The model under review builds one solid part; all positions refer to its coordinate system, in mm. Give positions to 0.01 mm unless a question says otherwise; leave off trailing zeros. Loops run counter-clockwise (first coordinate to the right, second up) from the corner with the lowest first, then second, coordinate; pieces in that order, holes last. Notation, with made-up numbers: (68, 22.5) - (98, 22.5) arc R19 ccw to (98, 43.5) - close; hole circle Ø5 at (-30, 88). An arc over 180 degrees is marked (long way). Return JSON: item names as keys, results as strings. Group by question number.
```python
from build123d import *

# Parameters (mm, degrees)
BOSS_EXTRUDE1_DEPTH   = 7
F_3_0MM_DOWEL_HOLE1_D = 3


with BuildPart() as part:
    # Sketch1 → Boss-Extrude1 (new body)
    with BuildSketch(Plane.XY):
        with BuildLine():
            ThreePointArc((0, 30), (-30, 0), (0, -30))
            ThreePointArc((0, -30), (5, -25), (0, -20))
            ThreePointArc((0, -20), (-20, 0), (0, 20))
            ThreePointArc((0, 20), (5, 25), (0, 30))
        make_face()
    extrude(amount=BOSS_EXTRUDE1_DEPTH)

    # Ø3.0mm Dowel Hole1 (through all)
    with Locations(Plane.XY.offset(7)):
        with Locations((0, 25), (0, -25)):
            Hole(F_3_0MM_DOWEL_HOLE1_D / 2)


solid = part.part
```
1) We need section D-D, the plane y = 17.5. Write out the cut boundary in (x, z).
2) We need section C-C, the plane y = 25. Write out the cut boundary in (x, z), plus the area to 3 significant figures.
3) For pin 1 Ø1 at (y, z) = (12.5, 4) entering from +X; pin 2 Ø2 at (x, z) = (-6, 6) entering from -Y; pin 3 Ø2 at (y, z) = (3.5, 3.5) entering from +X, all flat-tipped, find the tip position at first contact; note any pin that passes through.
4) We need section A-A, the plane z = 1.5. Write out the cut boundary in (x, y).
5) Draft analysis for pull direction Y (two halves, no side actions). For faces 1 (the face through (-29.993, 0.66, 3.451)), 2 (the face through (-21, 0, 7)), 3 (the face through (-20, 0, 3)), state which applies: +Y half, -Y half, draft (parallel to the pull), parting line (faces both ways), or undercut.
6) To check wall thickness, follow line 1 (Y direction, x = -10, z = 4.5); line 2 (Y direction, x = -16, z = 4.25); line 3 (Y direction, x = -24.5, z = 1). State the ranges of each line that lie inside material, in increasing order.
7) We need section B-B, the plane x = -16. Write out the cut boundary in (y, z).
Findings:
{
 "1": {"outline": "(-24.37, 0) - (-9.68, 0) - (-9.68, 7) - (-24.37, 7) - close"},
 "2": {"outline": "(-16.58, 0) - (-1.5, 0) - (-1.5, 7) - (-16.58, 7) - close; (1.5, 0) - (5, 0) - (5, 7) - (1.5, 7) - close", "area": "130 mm^2"},
 "3": {"pin 1": "stops at x = -15.2", "pin 2": "stops at y = -29.58", "pin 3": "stops at x = -19.49"},
 "4": {"outline": "(0, -30) arc R5 ccw to (0, -20) arc R20 cw to (0, 20) arc R5 ccw to (0, 30) arc R30 ccw to start; hole circle Ø3 at (0, -25); hole circle Ø3 at (0, 25)"},
 "5": {"face 1": "parting line", "face 2": "draft", "face 3": "undercut"},
 "6": {"line 1": "y = -28.28 to -17.32, 17.32 to 28.28", "line 2": "y = -25.38 to -12, 12 to 25.38", "line 3": "y = -17.31 to 17.31"},
 "7": {"outline": "(-25.38, 0) - (-12, 0) - (-12, 7) - (-25.38, 7) - close; (12, 0) - (25.38, 0) - (25.38, 7) - (12, 7) - close"}
}
